from build123d import *

# Parameters (mm, degrees)
CYLINDER_R         = 1.5
CYLINDER_DEPTH     = 13.3333
ARRAY_X_COUNT      = 2
ARRAY_X_PITCH      = 17
ARRAY_Y_COUNT      = 2
ARRAY_Y_PITCH      = 37
BOX021003019_W     = 25
BOX021003019_H     = 45
BOX021003019_DEPTH = 2


with BuildPart() as obj1:
    # Cylinder → Cylinder (new body)
    with BuildSketch(Plane(origin=(54, 54, 0), x_dir=(1, 0, 0), z_dir=(0, 0, 1))):
        Circle(CYLINDER_R)
    extrude(amount=CYLINDER_DEPTH)

    # Array X: obj1_2


with BuildPart() as obj1_1:
    add(obj1.part)
    with Locations(*[(i * ARRAY_X_PITCH, 0, 0) for i in range(1, ARRAY_X_COUNT)]):
        add(obj1.part)

    # Array Y: obj1_2


with BuildPart() as obj1_2:
    add(obj1_1.part)
    with Locations(*[(0, i * ARRAY_Y_PITCH, 0) for i in range(1, ARRAY_Y_COUNT)]):
        add(obj1_1.part)


with BuildPart() as mesa_sofa:
    # Box021003019 → Box021003019 (new body)
    with BuildSketch(Plane(origin=(50, 50, 13.3333), x_dir=(1, 0, 0), z_dir=(0, 0, 1))):
        with Locations((12.5, 22.5)):
            Rectangle(BOX021003019_W, BOX021003019_H)
    extrude(amount=BOX021003019_DEPTH)

    # Fusion009: union obj1
    add(obj1_2.part)


solid = mesa_sofa.part
Verification items for the finished model (mm, model axes). A direction names the side the tool comes from. Round coordinates to 2 decimals unless told otherwise and drop trailing zeros. Loops run counter-clockwise (first coordinate to the right, second up) from the corner with the lowest first, then second, coordinate; pieces in that order, holes last. Notation, with made-up numbers: (79.25, 42) - (90.25, 42) arc R20 cw to (90.25, 65) - close; hole circle Ø5 at (-26, 49.5). An arc over 180 degrees is marked (long way). Use a Markdown table: item, result. Add a question column.
1. Section check B-B, the plane y = 91. Record the boundary of the cut face in (x, z).
2. Section check A-A, the plane x = 71. Record the boundary of the cut face in (y, z), plus the area to 3 significant figures.
3. Thickness scan on probe 1 along Z at (x, y) = (68, 55.5); probe 2 along X at (y, z) = (55, 0.75). Record the ranges inside material, lowest first. Write a range as [from, to].
4. Section check D-D, the plane y = 65. Record the boundary of the cut face in (x, z).
5. Section check C-C, the plane z = 5. Record the boundary of the cut face in (x, y), plus the area to 3 significant figures.
6. Gauge pin test, flat ends, axial feed: pin 1 (12 mm diameter, centred on x = 69, y = 76.5, fed in from -Z); pin 2 (4 mm diameter, centred on x = 69, z = 4.5, fed in from +Y). Record the tip position at first contact, or that the pin passes through.
7. Access from +Z, -Z, +X, -X, +Y, -Y to the whole of each face (thin tool, end or side, straight path). Record for faces 1 (the face through (71.806, 92.265, 6.573)), 2 (the face through (71, 91, 0)).
8. Release check for a two-part mould opening along X. For faces 3 (the face through (54.69, 52.67, 6.57)), 4 (the face through (62, 73, 15.333)), 5 (the face through (75, 72, 14)) record: released by +X, released by -X, zero draft, split by the parting line, or undercut.
Checks:
| question | item | result |
|---|---|---|
| 1 | outline | (50, 13.33) - (52.5, 13.33) - (52.5, 0) - (55.5, 0) - (55.5, 13.33) - (69.5, 13.33) - (69.5, 0) - (72.5, 0) - (72.5, 13.33) - (75, 13.33) - (75, 15.33) - (50, 15.33) - close |
| 2 | outline | (50, 13.33) - (52.5, 13.33) - (52.5, 0) - (55.5, 0) - (55.5, 13.33) - (89.5, 13.33) - (89.5, 0) - (92.5, 0) - (92.5, 13.33) - (95, 13.33) - (95, 15.33) - (50, 15.33) - close |
| 2 | area | 170 mm^2 |
| 3 | probe 1 | z = [13.33, 15.33] |
| 3 | probe 2 | x = [52.88, 55.12], [69.88, 72.12] |
| 4 | outline | (50, 13.33) - (75, 13.33) - (75, 15.33) - (50, 15.33) - close |
| 5 | outline | circle Ø3 at (54, 54); circle Ø3 at (54, 91); circle Ø3 at (71, 54); circle Ø3 at (71, 91) |
| 5 | area | 28.3 mm^2 |
| 6 | pin 1 | stops at z = 13.33 |
| 6 | pin 2 | stops at y = 92.5 |
| 7 | face 1 | -Z |
| 7 | face 2 | -Z, +X, -X, +Y, -Y |
| 8 | face 3 | undercut |
| 8 | face 4 | zero draft |
| 8 | face 5 | released by +X |
